from build123d import *

# Parameters (mm, degrees)
F0_W     = 152.4
F0_H     = 63.5
F1_DEPTH = 76.2
F2_SIZE  = 25.4
F3_T     = -12.7


with BuildPart() as f1:
    # F0 (on Top) → F1 (new body)
    with BuildSketch(Plane.XY):
        with Locations((0, -13.890435)):
            Rectangle(F0_W, F0_H)
        Polygon((0, 85.793309), (-76.2, 17.859565), (76.2, 17.859565), align=None)
    extrude(amount=F1_DEPTH)

    # F2
    f2_edges = [f1.edges().sort_by_distance(p)[0] for p in [
        (0, -45.640435, 76.2),
    ]]
    chamfer(f2_edges, length=F2_SIZE)

    # F3
    f3_openings = [f1.faces().sort_by_distance(p)[0] for p in [
        (0, 5.065891, 0),
    ]]
    offset(amount=F3_T, openings=f3_openings)


solid = f1.part
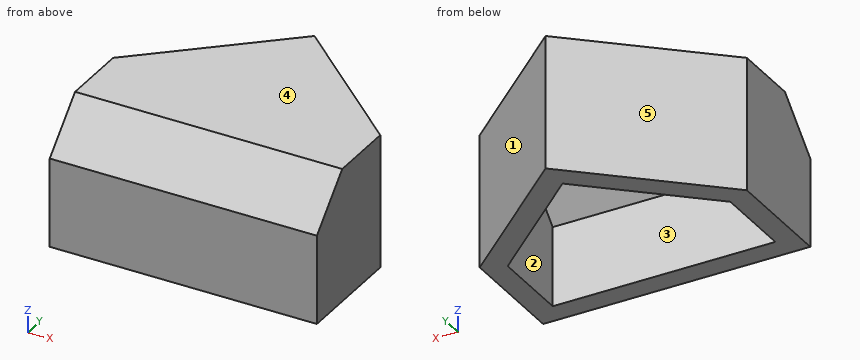
Geometry: final body of the model. Coordinates: model frame, mm. Face numbers are marked on the shaded views. A direction names the side the tool comes from. Coordinates: 2 decimals unless noted, no trailing zeros. Order: outer loops, then holes, each group sorted by start corner. A loop starts at its lowest first (then second) coordinate and runs counter-clockwise, first axis right, second up.
(1) Draft query along X for the marked faces 3, 4 and 5. Return one class per face: pulls with the +X half, pulls with the -X half, needs draft (parallel to the pull), parting line crosses it, or undercut.
(2) Material intervals for probe 1 along X at (y, z) = (-3, 21); probe 2 along Y at (x, z) = (62, 20.5); probe 3 along Y at (x, z) = (28, 35.5), sorted ascending.
(3) Access query for the marked faces 1 and 2. Directions: +Z, -Z, +X, -X, +Y, -Y. A direction counts if a zero-diameter tool reaches every point of the face in a straight line with its end or side. Return the directions, or none.
(4) First-contact query: pin 1 (5 mm diameter, centred on x = 34.5, z = 43.5, fed in from +Y); pin 2 (8 mm diameter, centred on x = 36, y = -22.5, fed in from -Z); pin 3 (5 mm diameter, centred on x = -14.5, y = -22.5, fed in from -Z). Flat tips, straight axial feed; report the tip coordinate or a pass-through.
(5) Section query B-B (y = -8). Return the cut outline in (x, z).
(6) Section query C-C (x = 14). Return the cut outline in (y, z), plus the area to 3 significant figures.
(7) Section query D-D (x = -42). Return the cut outline in (y, z), plus the area to 3 significant figures.
(8) Section query A-A (z = 36). Return the cut outline in (x, y).
Solution:
1. face 3: undercut
1. face 4: needs draft
1. face 5: pulls with the -X half
2. probe 1: x = -76.2 to -63.5, 63.5 to 76.2
2. probe 2: y = -45.64 to -32.94, 13.5 to 30.52
2. probe 3: y = -45.64 to -32.94, 43.82 to 60.83
3. face 1: +Z, -Z, +X, +Y
3. face 2: -Z
4. pin 1: stops at y = 57.26
4. pin 2: stops at z = 51.98
4. pin 3: stops at z = 53.48
5. outline: (-76.2, 0) - (-63.5, 0) - (-63.5, 63.5) - (63.5, 63.5) - (63.5, 0) - (76.2, 0) - (76.2, 76.2) - (-76.2, 76.2) - close
6. outline: (-45.64, 0) - (-32.94, 0) - (-32.94, 45.54) - (-14.98, 63.5) - (56.3, 63.5) - (56.3, 0) - (73.31, 0) - (73.31, 76.2) - (-20.24, 76.2) - (-45.64, 50.8) - close
6. area: 3,240 mm2
7. outline: (-45.64, 0) - (-32.94, 0) - (-32.94, 45.54) - (-14.98, 63.5) - (31.34, 63.5) - (31.34, 0) - (48.35, 0) - (48.35, 76.2) - (-20.24, 76.2) - (-45.64, 50.8) - close
7. area: 2,920 mm2
8. outline: (-76.2, -45.64) - (76.2, -45.64) - (76.2, 17.86) - (0, 85.79) - (-76.2, 17.86) - close; hole (-63.5, -32.94) - (63.5, -32.94) - (63.5, 12.17) - (0, 68.78) - (-63.5, 12.17) - close
